Part model, mm, in its own coordinate system. Face numbers are marked on the shaded views. A direction names the side the tool comes from. Give positions to 0.01 mm unless a question says otherwise; leave off trailing zeros. Write each loop counter-clockwise with the first axis right and the second up, starting at its lowest first coordinate (ties: lowest second). Pieces come first, ordered by that corner, then holes.
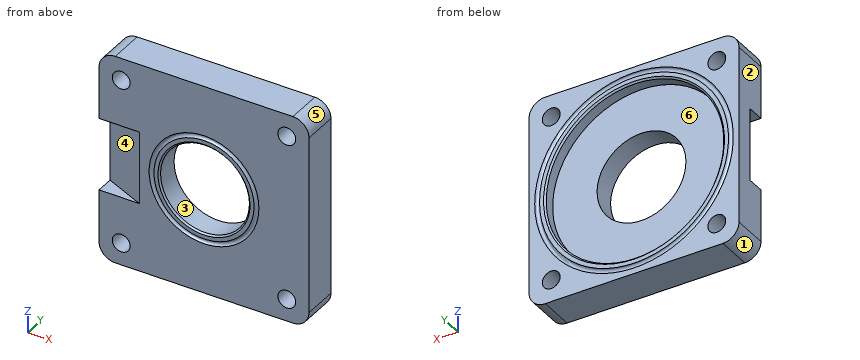
from build123d import *

# Parameters (mm, degrees)
SKETCH1_W           = 130
SKETCH1_H           = 130
SKETCH1_R           = 5.5
SKETCH1_R_2         = 27.5
BOSS_EXTRUDE1_DEPTH = 22
FILLET1_R           = 10
SKETCH2_R           = 55
CUT_EXTRUDE1_DEPTH  = 7.5
SKETCH4_R           = 1.5
CUT_EXTRUDE2_DEPTH  = 22.5
SKETCH8_R           = 1.5
CHAMFER1_SIZE       = 1


with BuildPart() as part:
    # Sketch1 → Boss-Extrude1 (new body)
    with BuildSketch(Plane(origin=(0, 0, 0), x_dir=(1, 0, 0), z_dir=(0, 1, 0))):
        Rectangle(SKETCH1_W, SKETCH1_H)
        with Locations(Location((51.265241636, 51.265241636, 0), (0, 0, 270))):
            Circle(SKETCH1_R, mode=Mode.SUBTRACT)
        with Locations(Location((-51.265241636, 51.265241636, 0), (0, 0, 270))):
            Circle(SKETCH1_R, mode=Mode.SUBTRACT)
        with Locations(Location((51.265241636, -51.265241636, 0), (0, 0, 270))):
            Circle(SKETCH1_R, mode=Mode.SUBTRACT)
        with Locations(Location((-51.265241636, -51.265241636, 0), (0, 0, 270))):
            Circle(SKETCH1_R, mode=Mode.SUBTRACT)
        with Locations(Location((0, 0, 0), (0, 0, 270))):
            Circle(SKETCH1_R_2, mode=Mode.SUBTRACT)
    extrude(amount=BOSS_EXTRUDE1_DEPTH)

    # Fillet1
    fillet1_edges = [part.edges().sort_by_distance(p)[0] for p in [
        (65, 11, 65),
        (-65, 11, 65),
        (-65, 11, -65),
        (65, 11, -65),
    ]]
    fillet(fillet1_edges, radius=FILLET1_R)

    # Sketch2 → Cut-Extrude1 (cut)
    with BuildSketch(Plane(origin=(0, 22, 0), x_dir=(1, 0, 0), z_dir=(0, 1, 0))):
        with Locations(Location((0, 0, 0), (0, 0, 270))):
            Circle(SKETCH2_R)
    extrude(amount=-CUT_EXTRUDE1_DEPTH, mode=Mode.SUBTRACT)

    # Cut-Sweep2: sweep along a path in Sketch3
    with BuildLine(Plane.XZ) as cut_sweep2_path:
        CenterArc((0, 0), 32.5, 0, 360)
    # Sketch4 → Cut-Sweep2 (sweep, cut)
    with BuildSketch(Plane.XY):
        with Locations((32.5, 0)):
            Circle(SKETCH4_R)
    sweep(path=cut_sweep2_path.line, mode=Mode.SUBTRACT)

    # Sketch6 → Cut-Extrude2 (cut, symmetric)
    with BuildSketch(Plane.XY):
        Polygon((-65, 0), (-40, 0), (-65, 11), align=None)
    extrude(amount=CUT_EXTRUDE2_DEPTH, both=True, mode=Mode.SUBTRACT)

    # Cut-Sweep3: sweep along a path in Sketch7
    with BuildLine(Plane(origin=(0, 22, 0), x_dir=(1, 0, 0), z_dir=(0, 1, 0))) as cut_sweep3_path:
        CenterArc((0, 0), 60, 0, 360)
    # Sketch8 → Cut-Sweep3 (sweep, cut)
    with BuildSketch(Plane.XY):
        with Locations((60, 22)):
            Circle(SKETCH8_R)
    sweep(path=cut_sweep3_path.line, mode=Mode.SUBTRACT)

    # Chamfer1
    chamfer1_edges = [part.edges().sort_by_distance(p)[0] for p in [
        (0, 0, -27.5),
        (0, 22, -55),
    ]]
    chamfer(chamfer1_edges, length=CHAMFER1_SIZE)


solid = part.part
1) Saw through at B-B (z = 0). Write the cut outline in (x, y).
Check result:
outline: (-65, 11) - (-40, 0) - (-34, 0) arc R1.5 cw to (-31, 0) - (-28.5, 0) - (-27.5, 1) - (-27.5, 14.5) - (-55, 14.5) - (-55, 21) - (-56, 22) - (-58.5, 22) arc R1.5 cw to (-61.5, 22) - (-65, 22) - close; (27.5, 1) - (28.5, 0) - (31, 0) arc R1.5 cw to (34, 0) - (65, 0) - (65, 22) - (61.5, 22) arc R1.5 cw to (58.5, 22) - (56, 22) - (55, 21) - (55, 14.5) - (27.5, 14.5) - close
2) Mould opens along Z. For the marked faces 1, 2 and 3 say: +Z half, -Z half, draft (parallel to the pull), parting line (faces both ways), or undercut.
Check result:
face 1: -Z half
face 2: draft
face 3: undercut
3) 3-axis set-ups, long thin cutter, end or side, ignore diameter. For the marked faces 4, 5 and 6: which of +Z, -Z, +X, -X, +Y, -Y reach the whole face in a straight line?
Check result:
face 4: -X, -Y
face 5: +Z, +X, +Y, -Y
face 6: +Y
4) Drill centre lines: L1, parallel to X at y = 13, z = -53.5; L2, parallel to Z at x = -14.5, y = 1; L3, parallel to X at y = 6.75, z = -50. Where is each one in solid material? Low to high.
Check result:
L1: x = -65 to -56.29, -46.24 to 46.24, 56.29 to 65
L2: z = -65 to -30.33, -27.83 to -23.37, 23.37 to 27.83, 30.33 to 65
L3: x = -65 to -56.62, -45.91 to 45.91, 56.62 to 65
5) Saw through at A-A (x = 0). Write the cut outline in (y, z), and give its area (3 significant figures).
Check result:
outline: (0, -65) - (22, -65) - (22, -61.5) arc R1.5 cw to (22, -58.5) - (22, -56) - (21, -55) - (14.5, -55) - (14.5, -27.5) - (1, -27.5) - (0, -28.5) - (0, -31) arc R1.5 cw to (0, -34) - close; (0, 28.5) - (1, 27.5) - (14.5, 27.5) - (14.5, 55) - (21, 55) - (22, 56) - (22, 58.5) arc R1.5 cw to (22, 61.5) - (22, 65) - (0, 65) - (0, 34) arc R1.5 cw to (0, 31) - close
area: 1,220 mm2
6) Saw through at D-D (z = 50.5). State how many separate pieces and enclosed holes the cut face has, and give its area (3 significant figures).
Check result:
separate pieces: 3
enclosed holes: 0
area: 2,040 mm2
7) Flat gauge pins, fed straight in: P1, Ø8, axis at x = 47, z = 38, coming from the +Y side; P2, Ø1, axis at x = 15, z = -46, coming from the +Y side. Where does each tip first touch, or does it go through?
Check result:
P1: stops at y = 22
P2: stops at y = 14.5
8) Saw through at C-C (y = 18.5). Write the cut outline in (x, z).
Check result:
outline: (-65, -55) arc R10 ccw to (-55, -65) - (55, -65) arc R10 ccw to (65, -55) - (65, 55) arc R10 ccw to (55, 65) - (-55, 65) arc R10 ccw to (-65, 55) - close; hole circle Ø11 at (-51.27, -51.27); hole circle Ø11 at (-51.27, 51.27); hole circle Ø110 at (0, 0); hole circle Ø11 at (51.27, -51.27); hole circle Ø11 at (51.27, 51.27)
